Geometry check sheet. Reference: drawing and pictorial views, mm from the part's lowest x, y, z. A direction names the side the tool comes from. Round coordinates to 2 decimals unless told otherwise and drop trailing zeros. Loops run counter-clockwise (first coordinate to the right, second up) from the corner with the lowest first, then second, coordinate; pieces in that order, holes last. Notation, with made-up numbers: (-20, -21.75) - (9, -21.75) arc R24 cw to (9, -0.75) - close; hole circle Ø2 at (71.25, 74). An arc over 180 degrees is marked (long way). Answer as CSV lines item,"result". Start each with the question number.
1) Access from +Z, -Z, +X, -X, +Y, -Y to the whole of each face (thin tool, end or side, straight path). Record for the marked faces 4 and 5.
2) Cross-section at D-D on y = 41. Record the boundary of the cut face in (x, z) (1 decimal), and give its area (3 significant figures).
3) Cross-section at C-C on x = 25.5. Record the boundary of the cut face in (y, z) (1 decimal).
4) Thickness scan on line 1 along X through (y, z) = (29.5, 9.5) (1 decimal); line 2 along X through (y, z) = (33, 9.5) (1 decimal); line 3 along Y through (x, z) = (50.5, 9.25) (1 decimal). Record the ranges inside material, lowest first.
5) Cross-section at B-B on y = 53. Record the boundary of the cut face in (x, z) (1 decimal).
6) Cross-section at A-A on z = 18.25. Record the boundary of the cut face in (x, y) (1 decimal).
7) Depth check by flat-ended pin: P1, Ø11.5, axis at x = 45, z = 17, coming from the -Y side; P2, Ø7.5, axis at y = 37.5, z = 8, coming from the -X side (1 decimal); P3, Ø8, axis at x = 13, z = 10, coming from the +Y side (1 decimal). Enter the tip coordinate at first touch or a pass-through.
8) Draft check along Y on the marked faces 1, 2 and 3. Enter one of: released by +Y, released by -Y, zero draft, split by the parting line, or undercut.
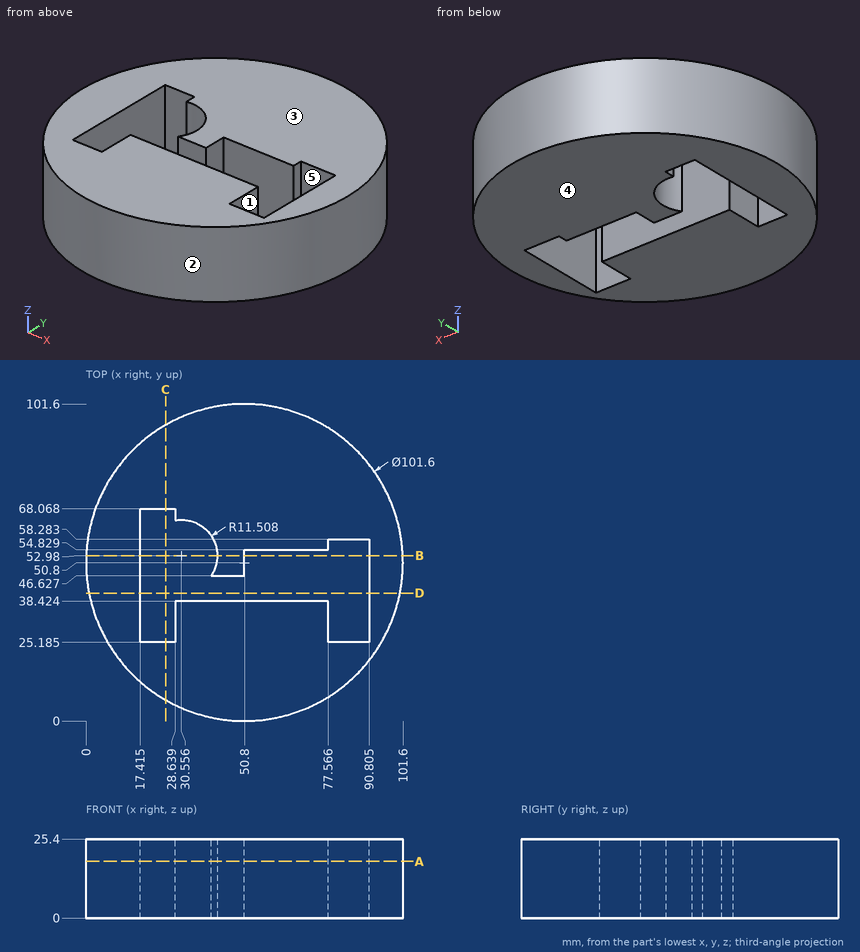
Answer block:
1,face 4,"-Z, +X, -X, +Y, -Y"
1,face 5,"+Z, -Z"
2,outline,"(1, 0) - (17.4, 0) - (17.4, 25.4) - (1, 25.4) - close; (90.8, 0) - (100.6, 0) - (100.6, 25.4) - (90.8, 25.4) - close"
2,area,"668 mm^2"
3,outline,"(6.7, 0) - (25.2, 0) - (25.2, 25.4) - (6.7, 25.4) - close; (68.1, 0) - (94.9, 0) - (94.9, 25.4) - (68.1, 25.4) - close"
4,line 1,"x = 4.7 to 17.4, 28.6 to 77.6, 90.8 to 96.9"
4,line 2,"x = 3.2 to 17.4, 28.6 to 77.6, 90.8 to 98.4"
4,line 3,"y = 0 to 38.4, 46.6 to 101.6"
5,outline,"(0, 0) - (17.4, 0) - (17.4, 25.4) - (0, 25.4) - close; (42.1, 0) - (50.8, 0) - (50.8, 25.4) - (42.1, 25.4) - close; (90.8, 0) - (101.6, 0) - (101.6, 25.4) - (90.8, 25.4) - close"
6,outline,"circle Ø101.6 at (50.8, 50.8); hole (17.4, 25.2) - (28.6, 25.2) - (28.6, 38.4) - (77.6, 38.4) - (77.6, 25.2) - (90.8, 25.2) - (90.8, 58.3) - (77.6, 58.3) - (77.6, 54.8) - (50.8, 54.8) - (50.8, 46.6) - (40.2, 46.6) arc R11.5 ccw to (28.6, 64.3) - (28.6, 68.1) - (17.4, 68.1) - close"
7,P1,"stops at y = 0"
7,P2,"stops at x = 0.9"
7,P3,"stops at y = 88.7"
8,face 1,"undercut"
8,face 2,"split by the parting line"
8,face 3,"zero draft"
